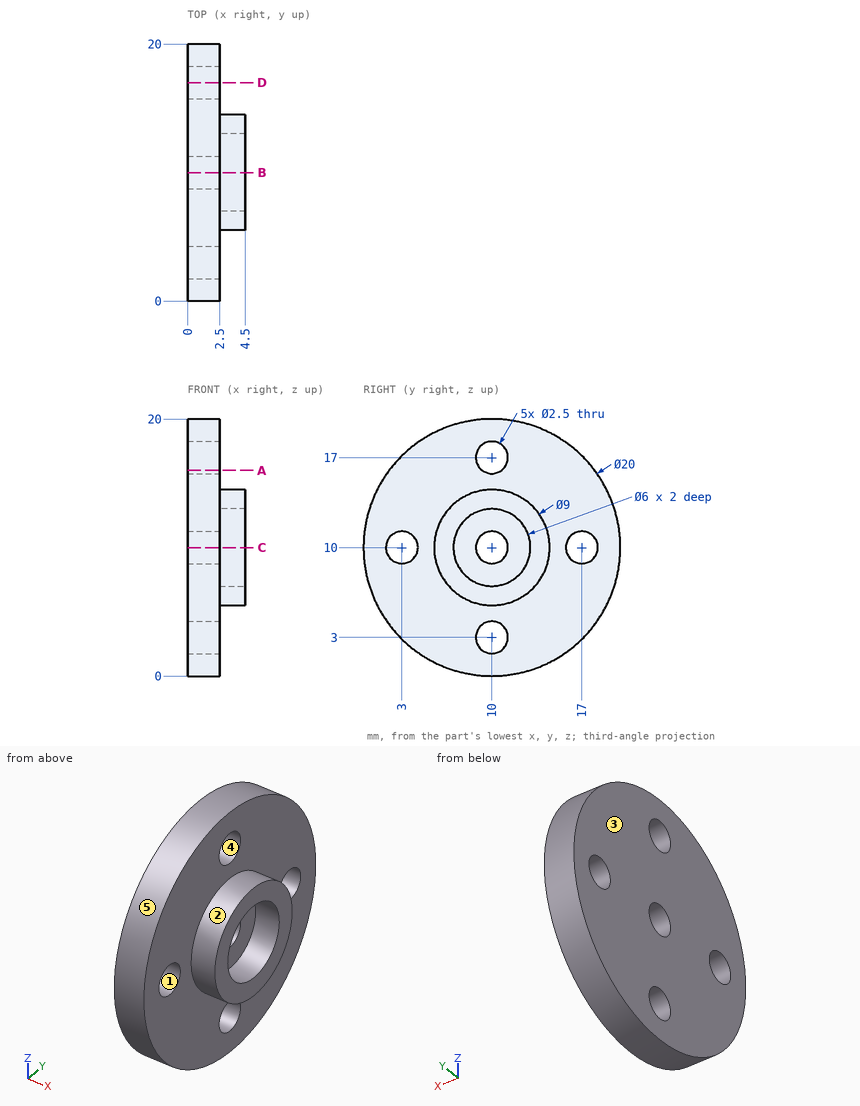
Study the drawing (mm; zero at the part's minimum x, y, z) and answer. A direction names the side the tool comes from. Give positions to 0.01 mm unless a question says otherwise; leave off trailing zeros. Loops run counter-clockwise (first coordinate to the right, second up) from the corner with the lowest first, then second, coordinate; pieces in that order, holes last. Notation, with made-up numbers: (82.25, -26) - (114.25, -26) arc R20 ccw to (114.25, -6) - close; hole circle Ø10 at (20.25, 64.5). An arc over 180 degrees is marked (long way). Return JSON: item names as keys, results as strings. Group by question number.
1. Find section D-D (y = 17). Write down the section's boundary in (x, z), then the cut area to 3 significant figures.
2. Find section B-B (y = 10). Write down the section's boundary in (x, z).
3. Find section A-A (z = 16). Write down the section's boundary in (x, y).
4. Given pin 1 Ø2 at (y, z) = (10, 17) entering from -X; pin 2 Ø1.5 at (x, y) = (2.5, 7.5) entering from -Z; pin 3 Ø1.5 at (x, z) = (3, 8.5) entering from -Y; pin 4 Ø1 at (x, y) = (2, 8) entering from -Z, each flat-ended and moving along its own axis, determine where each tip first touches the part or whether it passes through.
5. Straight lines are drawn through the part: line 1 (Y direction, x = 1.2, z = 10); line 2 (Y direction, x = 2, z = 9.25); line 3 (X direction, y = 4, z = 8). For each, find the intervals that lie inside material, in ascending order. Write a range as [from, to].
6. Which of the six approach directions +Z, -Z, +X, -X, +Y, -Y give full straight-line access (tool end or side, diameter ignored) to the marked faces 1 and 2?
7. Determine the mould class of the marked faces 3, 4 and 5 for opening direction Y: pulls with the +Y half, pulls with the -Y half, needs draft (parallel to the pull), parting line crosses it, or undercut.
Verdict:
{
 "1": {"outline": "(0, 2.86) - (2.5, 2.86) - (2.5, 8.75) - (0, 8.75) - close; (0, 11.25) - (2.5, 11.25) - (2.5, 17.14) - (0, 17.14) - close", "area": "29.5 mm^2"},
 "2": {"outline": "(0, 0) - (2.5, 0) - (2.5, 1.75) - (0, 1.75) - close; (0, 4.25) - (2.5, 4.25) - (2.5, 5.5) - (4.5, 5.5) - (4.5, 7) - (2.5, 7) - (2.5, 8.75) - (0, 8.75) - close; (0, 11.25) - (2.5, 11.25) - (2.5, 13) - (4.5, 13) - (4.5, 14.5) - (2.5, 14.5) - (2.5, 15.75) - (0, 15.75) - close; (0, 18.25) - (2.5, 18.25) - (2.5, 20) - (0, 20) - close"},
 "3": {"outline": "(0, 2) - (2.5, 2) - (2.5, 9.25) - (0, 9.25) - close; (0, 10.75) - (2.5, 10.75) - (2.5, 18) - (0, 18) - close"},
 "4": {"pin 1": "passes through", "pin 2": "stops at z = 0.15", "pin 3": "stops at y = 0.04", "pin 4": "stops at z = 0.11"},
 "5": {"line 1": "y = [0, 1.75], [4.25, 8.75], [11.25, 15.75], [18.25, 20]", "line 2": "y = [0.03, 2], [4, 9], [11, 16], [18, 19.97]", "line 3": "x = [0, 2.5]"},
 "6": {"face 1": "+X, -X", "face 2": "+X"},
 "7": {"face 3": "needs draft", "face 4": "undercut", "face 5": "parting line crosses it"}
}
